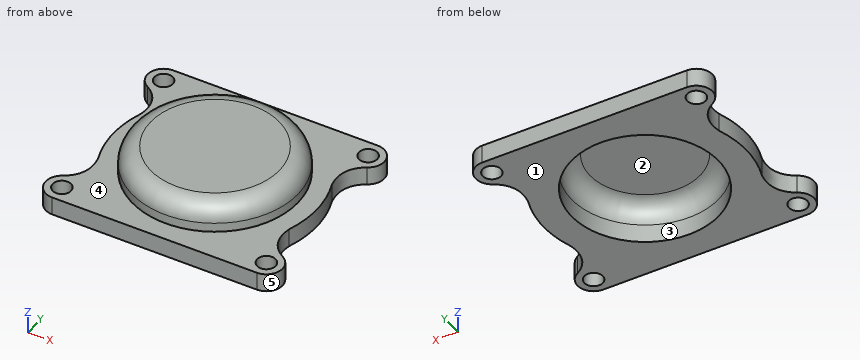
from build123d import *

# Parameters (mm, degrees)
SKETCH1_R           = 1
SKETCH1_R_2         = 7.975
BOSS_EXTRUDE1_DEPTH = 2
SKETCH2_R           = 8.975
SKETCH2_R_2         = 7.975
BOSS_EXTRUDE2_DEPTH = 2
SKETCH3_R           = 8.975
BOSS_EXTRUDE3_DEPTH = 1
FILLET1_R           = 2


with BuildPart() as part:
    # Sketch1 → Boss-Extrude1 (new body)
    with BuildSketch(Plane.XY):
        with BuildLine():
            Line((-10.866636256, -11.400091233), (11.133363744, -11.400091233))
            ThreePointArc((11.133363744, -11.400091233), (12.832206534, -10.070130727), (11.948884962, -8.101729149))
            add(Edge.make_bspline(
                [(11.948884962, -8.101729149), (9.883447826, -6.844292891), (10.420778008, -4.294845111)],
                knots=[0, 0, 0, 1, 1, 1], degree=2))
            ThreePointArc((10.420778008, -4.294845111), (11.133363745, -0.400091249), (10.420778018, 3.494662613))
            add(Edge.make_bspline(
                [(10.420778018, 3.494662613), (9.883447814, 6.044110418), (11.948884963, 7.301546684)],
                knots=[0, 0, 0, 1, 1, 1], degree=2))
            ThreePointArc((11.948884963, 7.301546684), (12.832206534, 9.269948262), (11.133363744, 10.599908767))
            Line((11.133363744, 10.599908767), (-10.866636256, 10.599908767))
            ThreePointArc((-10.866636256, 10.599908767), (-12.565479045, 9.269948261), (-11.682157474, 7.301546683))
            add(Edge.make_bspline(
                [(-11.682157474, 7.301546683), (-9.616720338, 6.044110425), (-10.15405052, 3.494662645)],
                knots=[0, 0, 0, 1, 1, 1], degree=2))
            ThreePointArc((-10.15405052, 3.494662645), (-10.866636257, -0.400091216), (-10.15405053, -4.294845078))
            add(Edge.make_bspline(
                [(-10.15405053, -4.294845078), (-9.616720326, -6.844292883), (-11.682157475, -8.101729149)],
                knots=[0, 0, 0, 1, 1, 1], degree=2))
            ThreePointArc((-11.682157475, -8.101729149), (-12.565479045, -10.070130727), (-10.866636256, -11.400091233))
        make_face()
        with Locations((-10.866636256, -9.650091233)):
            Circle(SKETCH1_R, mode=Mode.SUBTRACT)
        with Locations((11.133363744, -9.650091233)):
            Circle(SKETCH1_R, mode=Mode.SUBTRACT)
        with Locations((-10.866636256, 8.849908767)):
            Circle(SKETCH1_R, mode=Mode.SUBTRACT)
        with Locations((11.133363744, 8.849908767)):
            Circle(SKETCH1_R, mode=Mode.SUBTRACT)
        with Locations((0.133363744, -0.400091233)):
            Circle(SKETCH1_R_2, mode=Mode.SUBTRACT)
    extrude(amount=BOSS_EXTRUDE1_DEPTH)

    # Sketch2 → Boss-Extrude2 (add)
    with BuildSketch(Plane.XY.offset(2)):
        with Locations((0.133363744, -0.400091233)):
            Circle(SKETCH2_R)
        with Locations((0.133363744, -0.400091233)):
            Circle(SKETCH2_R_2, mode=Mode.SUBTRACT)
    extrude(amount=BOSS_EXTRUDE2_DEPTH)

    # Sketch3 → Boss-Extrude3 (add)
    with BuildSketch(Plane.XY.offset(4)):
        with Locations((0.133363744, -0.400091233)):
            Circle(SKETCH3_R)
    extrude(amount=BOSS_EXTRUDE3_DEPTH)

    # Fillet1
    fillet1_edges = [part.edges().sort_by_distance(p)[0] for p in [
        (-8.841636256, -0.400091233, 5),
        (-7.841636256, -0.400091233, 4),
    ]]
    fillet(fillet1_edges, radius=FILLET1_R)


solid = part.part
For this review, take the finished solid that the model builds, in its own axes (mm). Face numbers are marked on the shaded views. A direction names the side the tool comes from. Coordinates: 2 decimals unless noted, no trailing zeros. Loops run counter-clockwise (first coordinate to the right, second up) from the corner with the lowest first, then second, coordinate; pieces in that order, holes last. Notation, with made-up numbers: (84, 55.25) - (89, 55.25) arc R21 cw to (89, 63.25) - close; hole circle Ø6 at (14, 32.25). An arc over 180 degrees is marked (long way). Use a Markdown table: item, result. Add a question column.
Item 1: Mouldability with a two-part tool opening along X and no side actions: class the marked faces 3, 4 and 5 as pulls with the +X half, pulls with the -X half, needs draft (parallel to the pull), parting line crosses it, or undercut.
Item 2: For line 1 (Z direction, x = 10.25, y = 1.75); line 2 (Z direction, x = 2, y = -0.25); line 3 (X direction, y = 1, z = 3.45), list the stretches that pass through material, from the lowest coordinate up.
Item 3: We need section B-B (z = 4.3). Give the boundary of the cut face in (x, y).
Item 4: We need section A-A (x = -9.5). Give the boundary of the cut face in (y, z).
Item 5: Insertion check: pin 1 Ø13 at (x, y) = (0.13, -0.4) entering from -Z; pin 2 Ø1.2 at (x, y) = (11.13, -9.65) entering from -Z; pin 3 Ø3.5 at (x, y) = (-1.5, -1) entering from -Z; pin 4 Ø2 at (y, z) = (-6.5, 2.5) entering from +X. Each pin has a flat end and moves straight along its axis. Give the tip position at first contact, or say it passes through.
Item 6: Tool access review of the marked faces 1 and 2: name each direction out of +Z, -Z, +X, -X, +Y, -Y from which nothing blocks a thin tool from reaching the whole face with its end or side.
Item 7: We need section C-C (z = 0.6). Give the number of separate pieces and of enclosed holes in the cut face, and give its area (3 significant figures).
Results list:
| question | item | result |
|---|---|---|
| 1 | face 3 | undercut |
| 1 | face 4 | needs draft |
| 1 | face 5 | pulls with the +X half |
| 2 | line 1 | z = 0 to 2 |
| 2 | line 2 | z = 4 to 5 |
| 2 | line 3 | x = -8.68 to -7.08, 7.35 to 8.95 |
| 3 | outline | circle Ø16.99 at (0.13, -0.4) |
| 4 | outline | (-11.4, 0) - (10.6, 0) - (10.6, 2) - (-11.4, 2) - close |
| 5 | pin 1 | stops at z = 3.93 |
| 5 | pin 2 | passes through |
| 5 | pin 3 | stops at z = 4 |
| 5 | pin 4 | stops at x = 11.06 |
| 6 | face 1 | -Z, +X, -X, +Y, -Y |
| 6 | face 2 | -Z |
| 7 | separate pieces | 1 |
| 7 | enclosed holes | 5 |
| 7 | area | 280 mm^2 |
